Can you work these out from the drawing? Everything is in mm from the part's minimum corner. A direction names the side the tool comes from. Round coordinates to 2 decimals unless told otherwise and drop trailing zeros. Order: outer loops, then holes, each group sorted by start corner. A loop starts at its lowest first (then second) coordinate and runs counter-clockwise, first axis right, second up. Notation, with made-up numbers: (-25.75, -12) -> (-19.75, -12) arc R29 ccw to (-19.75, 23) -> close; hole circle Ø1 at (-3, -22). An arc over 180 degrees is marked (long way). Use a Markdown table: item, result. Add a question column.
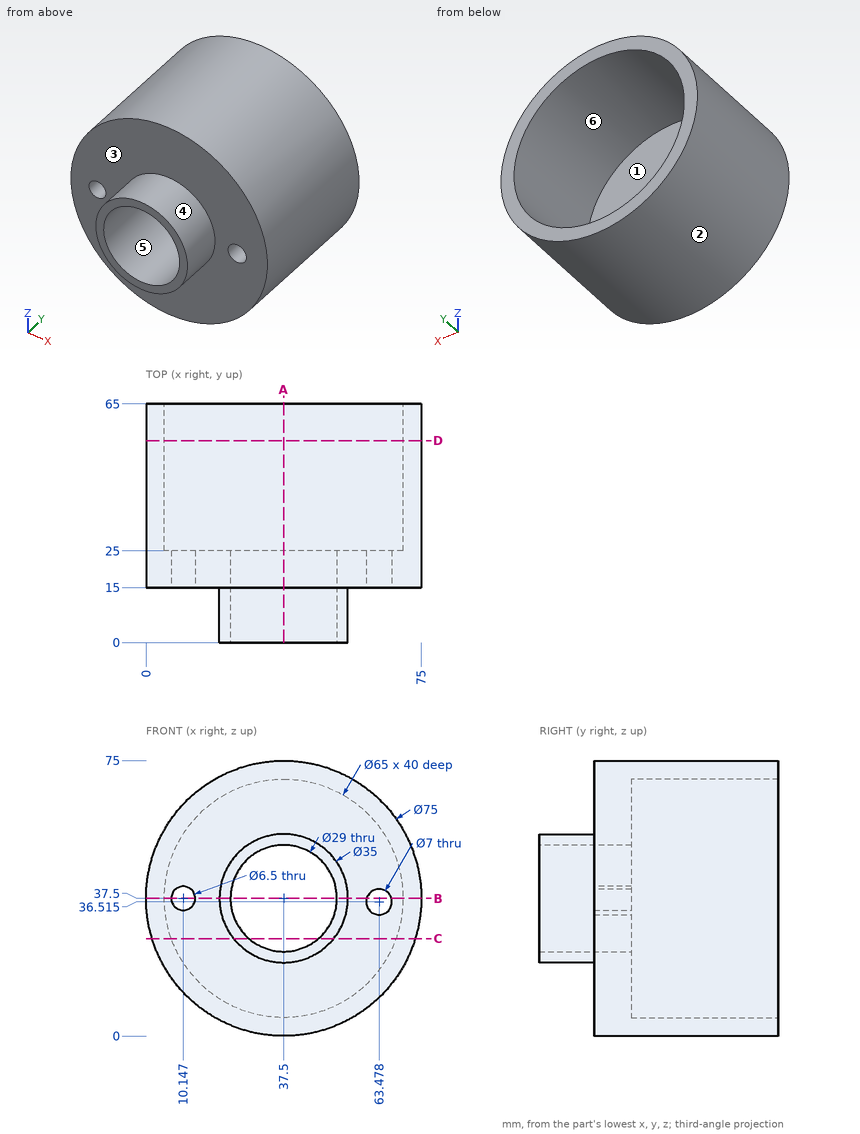
(1) I'm going to push flat-ended pins straight in: P1, Ø1, axis at x = 55.5, z = 29.5, coming from the +Y side; P2, Ø5, axis at x = 52.5, y = 53.5, coming from the -Z side (1 decimal); P3, Ø1.5, axis at x = 21, z = 60, coming from the -Y side; P4, Ø6.5, axis at x = 63.48, z = 36.52, coming from the -Y side. Where does each tip first touch, or does it pass through?
(2) I want a section at C-C on z = 26.5. List the corners of the cut face in (x, y) for me.
(3) If we mould it in two halves opening along Z, with no side actions, what happens to the marked faces 1, 2 and 3? For each: pulls with the +Z half, pulls with the -Z half, needs draft (parallel to the pull), parting line crosses it, or undercut.
(4) I want a section at B-B on z = 37.5. List the corners of the cut face in (x, y) for me.
(5) On a 3-axis mill with a long thin cutter (end or side, diameter ignored), from which of +Z, -Z, +X, -X, +Y, -Y can I reach the whole of each face in a straight line? I mean the marked faces 4, 5 and 6. Say none if no direction works.
(6) I want a section at D-D on y = 55. List the corners of the cut face in (x, z) for me.
(7) I want a section at A-A on x = 37.5. List the corners of the cut face in (y, z) for me, and give its area (3 significant figures).
(8) Please list where these lines run through material, in increasing order: probe 1 along X at (y, z) = (49, 37.5); probe 2 along X at (y, z) = (18.75, 37.5); probe 3 along Y at (x, z) = (19, 61.5). Write a range as from..to.
Output:
| question | item | result |
|---|---|---|
| 1 | P1 | y = 25 |
| 1 | P2 | z = 2.1 |
| 1 | P3 | y = 15 |
| 1 | P4 | through |
| 2 | outline | (1.65, 15) -> (23.89, 15) -> (23.89, 0) -> (28.05, 0) -> (28.05, 25) -> (6.92, 25) -> (6.92, 65) -> (1.65, 65) -> close; (46.95, 0) -> (51.11, 0) -> (51.11, 15) -> (73.35, 15) -> (73.35, 65) -> (68.08, 65) -> (68.08, 25) -> (46.95, 25) -> close |
| 3 | face 1 | undercut |
| 3 | face 2 | parting line crosses it |
| 3 | face 3 | needs draft |
| 4 | outline | (0, 15) -> (6.9, 15) -> (6.9, 25) -> (5, 25) -> (5, 65) -> (0, 65) -> close; (13.4, 15) -> (20, 15) -> (20, 0) -> (23, 0) -> (23, 25) -> (13.4, 25) -> close; (52, 0) -> (55, 0) -> (55, 15) -> (60.12, 15) -> (60.12, 25) -> (52, 25) -> close; (66.84, 15) -> (75, 15) -> (75, 65) -> (70, 65) -> (70, 25) -> (66.84, 25) -> close |
| 5 | face 4 | -Y |
| 5 | face 5 | +Y, -Y |
| 5 | face 6 | +Y |
| 6 | outline | circle Ø75 at (37.5, 37.5); hole circle Ø65 at (37.5, 37.5) |
| 7 | outline | (0, 20) -> (15, 20) -> (15, 0) -> (65, 0) -> (65, 5) -> (25, 5) -> (25, 23) -> (0, 23) -> close; (0, 52) -> (25, 52) -> (25, 70) -> (65, 70) -> (65, 75) -> (15, 75) -> (15, 55) -> (0, 55) -> close |
| 7 | area | 950 mm² |
| 8 | probe 1 | 0..5, 70..75 |
| 8 | probe 2 | 0..6.9, 13.4..23, 52..60.12, 66.84..75 |
| 8 | probe 3 | 15..25 |
